Geometry check sheet. Reference: the model listing, model coordinates, mm. Round coordinates to 2 decimals unless told otherwise and drop trailing zeros. Order: outer loops, then holes, each group sorted by start corner. A loop starts at its lowest first (then second) coordinate and runs counter-clockwise, first axis right, second up.
(1) Gauge pin test, flat end, axial feed: P1, Ø2.5, axis at x = 41, y = 0, coming from the +Z side. Record the tip position at first contact, or that the pin passes through.
(2) Cross-section at A-A on z = 0.4. Enter the section's corners in (x, y).
(3) Cross-section at B-B on x = -57. Enter the section's corners in (y, z), and give its area (3 significant figures).
(4) Thickness scan on L1, parallel to X at y = 71, z = 0.35; L2, parallel to Y at x = 41, z = -0.4; L3, parallel to Y at x = -41, z = 0.1. Record the ranges inside material, lowest first.
(5) Cross-section at C-C on y = -56. Enter the section's corners in (x, z).
Autodesk Inventor part; units mm, degrees
sketch "Эскиз1" plane through (0, 0, 0) normal (0, 0, 1) x (1, 0, 0)
  line L0 (-45, -75) -> (45, -75)
  line L1 (45, -75) -> (45, 75)
  line L2 (45, 75) -> (-85, 75)
  line L3 (-45, 0) -> (-45, -75)
  line L4 (-45, -75) -> (45, 75) construction
  line L5 (45, -75) -> (-45, 75) construction
  line L6 (-85, 75) -> (-85, 0)
  line L7 (-85, 0) -> (-49.5, 0)
  line L8 (-45, 0) -> (-85, 0)
  line L9 (-45, -5) -> (-85, 35)
  point P0 (0, 0)
  dimension "d0" = 90
  dimension "d1" = 150
  dimension "d22" = 75
  dimension "d25" = 130
  dimension "d26" = 45
  dimension "d27" = 40
extrude "Выдавливание1" add sketch "Эскиз1" along normal mid plane 2 contours L3 L8 L7 L9 L6 L2 L1 L0 | L9 L7 L8 L3
fillet "Сопряжение2" radius 4 6 edges at (45, 75, 0) (45, -75, 0) (-45, -75, 0) (-45, -5, 0) (-85, 35, 0) (-85, 75, 0)
sketch "Эскиз4" plane through (0, 0, 1) normal (0, 0, 1) x (1, 0, 0)
  circle A0 centre (-81, 36.6569) radius 1.5
  circle A1 centre (-41, 0) radius 1.5
  circle A2 centre (41, 0) radius 1.5
  circle A3 centre (41, -71) radius 1.5
  circle A4 centre (-41, -71) radius 1.5
  circle A5 centre (41, 71) radius 1.5
  circle A6 centre (-81, 71) radius 1.5
  arc A7 (-81, 75) -> (-85, 71) centre (-81, 71) ccw construction
  line L0 (-85, 71) -> (-85, 36.6569) construction
  arc A8 (-85, 36.6569) -> (-83.8284, 33.8284) centre (-81, 36.6569) ccw construction
  line L1 (-83.8284, 33.8284) -> (-46.1716, -3.8284) construction
  arc A9 (-45, -6.6569) -> (-46.1716, -3.8284) centre (-49, -6.6569) ccw construction
  line L2 (-45, -6.6569) -> (-45, -71) construction
  arc A10 (-45, -71) -> (-41, -75) centre (-41, -71) ccw construction
  line L3 (-41, -75) -> (41, -75) construction
  arc A11 (41, -75) -> (45, -71) centre (41, -71) ccw construction
  line L4 (45, -71) -> (45, 71) construction
  arc A12 (45, 71) -> (41, 75) centre (41, 71) ccw construction
  line L5 (41, 75) -> (-81, 75) construction
  line L6 (-81, 71) -> (-81, 36.6569) construction
  line L7 (-81, 36.6569) -> (-43.3431, -1) construction
  arc A13 (-41, -6.6569) -> (-43.3431, -1) centre (-49, -6.6569) ccw construction
  line L8 (-41, -6.6569) -> (-41, -71) construction
  line L9 (-41, -71) -> (41, -71) construction
  line L10 (41, -71) -> (41, 71) construction
  line L11 (41, 71) -> (-81, 71) construction
  line L12 (-112.1598, 0) -> (72.1598, 0)
  point P0 (0, 0)
  point P1 (41, 0)
  dimension "d29" = 3
  dimension "d30" = 4
  dimension "d31" = 41
extrude "Выдавливание4" cut sketch "Эскиз4" against normal through all
properties part number "Контур платы"
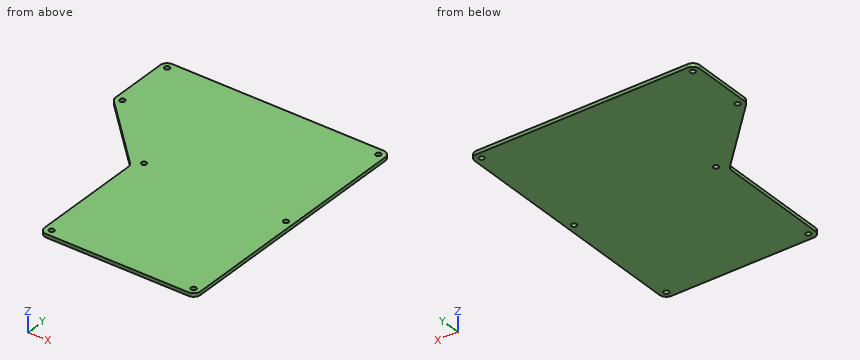
Found:
1. P1: passes through
2. outline: (-85, 36.66) arc R4 ccw to (-83.83, 33.83) - (-46.17, -3.83) arc R4 cw to (-45, -6.66) - (-45, -71) arc R4 ccw to (-41, -75) - (41, -75) arc R4 ccw to (45, -71) - (45, 71) arc R4 ccw to (41, 75) - (-81, 75) arc R4 ccw to (-85, 71) - close; hole circle Ø3 at (-81, 36.66); hole circle Ø3 at (-81, 71); hole circle Ø3 at (-41, -71); hole circle Ø3 at (-41, 0); hole circle Ø3 at (41, -71); hole circle Ø3 at (41, 0); hole circle Ø3 at (41, 71)
3. outline: (7, -1) - (75, -1) - (75, 1) - (7, 1) - close
3. area: 136 mm2
4. L1: x = -85 to -82.5, -79.5 to 39.5, 42.5 to 45
4. L2: y = -75 to -72.5, -69.5 to -1.5, 1.5 to 69.5, 72.5 to 75
4. L3: y = -75 to -72.5, -69.5 to -1.5, 1.5 to 75
5. outline: (-45, -1) - (45, -1) - (45, 1) - (-45, 1) - close
